```python
from build123d import *

# Parameters (mm, degrees)
F0_W     = 600
F0_H     = 150
F1_DEPTH = 22
F2_D     = 6.6
F3_D     = 5.5
F4_D     = 26
F5_D     = 4.5


with BuildPart() as f1:
    # F0 (on Top) → F1 (new body)
    with BuildSketch(Plane.XY):
        with Locations((269.0510096401, 81.4705566212)):
            Rectangle(F0_W, F0_H)
    extrude(amount=F1_DEPTH)

    # F2 (through all)
    with Locations(Plane(origin=(0, 0, 0), x_dir=(1, 0, 0), z_dir=(0, 0, -1))):
        with Locations((499.0510096401, -113.9705566212), (534.0510096401, -113.9705566212), (499.0510096401, -148.9705566212), (534.0510096401, -148.9705566212), (534.0510096401, -13.9705566212), (499.0510096401, -48.9705566212), (499.0510096401, -13.9705566212), (534.0510096401, -48.9705566212)):
            Hole(F2_D / 2)

    # F3 (through all)
    with Locations(Plane(origin=(0, 0, 0), x_dir=(1, 0, 0), z_dir=(0, 0, -1))):
        with Locations((-15.9489903599, -21.4705566212), (14.0510096401, -21.4705566212), (104.0510096401, -51.4705566212), (104.0510096401, -21.4705566212), (14.0510096401, -51.4705566212), (134.0510096401, -51.4705566212), (134.0510096401, -21.4705566212), (-15.9489903599, -51.4705566212)):
            Hole(F3_D / 2)

    # F4 (through all)
    with Locations(Plane(origin=(0, 0, 0), x_dir=(1, 0, 0), z_dir=(0, 0, -1))):
        with Locations((59.0510096401, -81.4705566212)):
            Hole(F4_D / 2)

    # F5 (through all)
    with Locations(Plane(origin=(0, 0, 0), x_dir=(1, 0, 0), z_dir=(0, 0, -1))):
        with Locations((561.5510096401, -113.9705566212), (561.5510096401, -48.9705566212)):
            Hole(F5_D / 2)


solid = f1.part
```
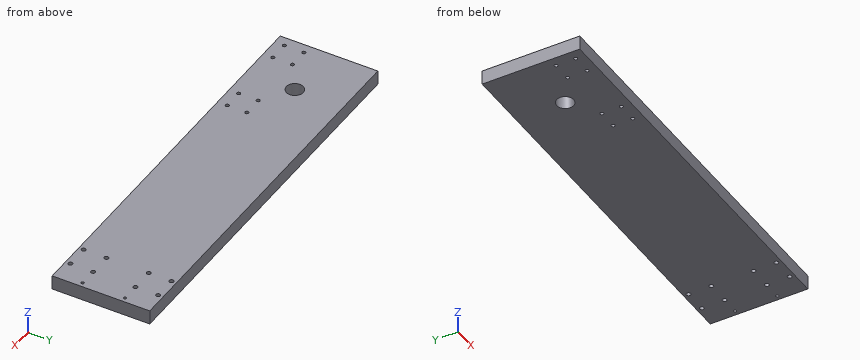
Check sheet for the modelled part. Datum: model origin and axes. Units: mm. Round coordinates to 2 decimals unless told otherwise and drop trailing zeros. Loops run counter-clockwise (first coordinate to the right, second up) from the corner with the lowest first, then second, coordinate; pieces in that order, holes last. Notation, with made-up numbers: M 84.5,43 L 92.5,43 A16 ccw 92.5,63 Z; hole C 66.5,-12.5 d3. An arc over 180 degrees is marked long. Answer as a JSON object with one key per item and string values.
1. Scan lines: line 1 (X direction, y = 17, z = 15.5); line 2 (X direction, y = 116.5, z = 11); line 3 (X direction, y = 71.5, z = 16.25). Record each from-to range of solid material in increasing order.
Reply:
{"line 1": "x = -30.95 to 497.74, 500.36 to 532.74, 535.36 to 569.05", "line 2": "x = -30.95 to 496.93, 501.17 to 531.93, 536.17 to 569.05", "line 3": "x = -30.95 to 50.71, 67.39 to 569.05"}
2. Section check A-A (y = 76.5). Record the boundary of the cut face in (x, z), plus the area to 3 significant figures.
Reply:
{"outline": "M -30.95,0 L 47.04,0 L 47.04,22 L -30.95,22 Z; M 71.06,0 L 569.05,0 L 569.05,22 L 71.06,22 Z", "area": "12,700 mm²"}
3. Gauge pin test, flat end, axial feed: P1, Ø4.5, axis at x = 14.05, y = 51.47, coming from the +Z side. Record the tip position at first contact, or that the pin passes through.
Reply:
{"P1": "passes through"}
